```python
from build123d import *

# Parameters (mm, degrees)
RESSALTO_EXTRUS_O1_DEPTH            = 3
ESCAREADO_PARA_SFHCS_M31_AT_2_COUNT = 2
ESCAREADO_PARA_SFHCS_M31_AT_2_PITCH = 117.96437389
ESCAREADO_PARA_SFHCS_M31_AT_3_COUNT = 2
ESCAREADO_PARA_SFHCS_M31_AT_3_PITCH = 80
ESCAREADO_PARA_SFHCS_M31_AT_4_COUNT = 2
ESCAREADO_PARA_SFHCS_M31_AT_4_PITCH = 156.207361139
FILETE1_R                           = 4


with BuildPart() as part:
    # Esboço1 → Ressalto-extrusão1 (new body)
    with BuildSketch(Plane(origin=(0, 0, 0), x_dir=(1, 0, 0), z_dir=(0, 1, 0))):
        with BuildLine():
            Line((-68.089865002, 52.533515816), (-60.990156529, 50.415201884))
            Line((-60.990156529, 50.415201884), (-51.474506905, 61.094962266))
            Line((-51.474506905, 61.094962266), (-51.366345618, 68.974622419))
            ThreePointArc((-51.366345618, 68.974622419), (0, 86), (51.366345618, 68.974622419))
            Line((51.366345618, 68.974622419), (51.474506905, 61.094962266))
            Line((51.474506905, 61.094962266), (60.990156529, 50.415201884))
            Line((60.990156529, 50.415201884), (68.089865002, 52.533515816))
            ThreePointArc((68.089865002, 52.533515816), (85.999638052, 0.24950947), (68.393545574, -52.137538529))
            Line((68.393545574, -52.137538529), (60.990156529, -51.512941417))
            Line((60.990156529, -51.512941417), (50.318654012, -60.477268457))
            Line((50.318654012, -60.477268457), (51.474506905, -68.893941235))
            ThreePointArc((51.474506905, -68.893941235), (44.026252256, -73.876174185), (36.1, -78.056325817))
            Line((36.1, -78.056325817), (-36.1, -78.056325817))
            ThreePointArc((-36.1, -78.056325817), (-44.026252256, -73.876174185), (-51.474506905, -68.893941235))
            Line((-51.474506905, -68.893941235), (-50.318654012, -60.477268457))
            Line((-50.318654012, -60.477268457), (-60.990156529, -51.512941417))
            Line((-60.990156529, -51.512941417), (-68.393545574, -52.137538529))
            ThreePointArc((-68.393545574, -52.137538529), (-85.999638052, 0.24950947), (-68.089865002, 52.533515816))
        make_face()
    extrude(amount=RESSALTO_EXTRUS_O1_DEPTH)

    # Esboço3 → Escareado para SFHCS M31 (revolve, cut)
    with BuildSketch(Plane(origin=(40, 3, 69.282032303), x_dir=(0, 0, 1), z_dir=(1, 0, 0))):
        Polygon((0, 0), (0, 3), (1.7, 3), (1.7, 1.66), (3.36, 0), align=None)
    escareado_para_sfhcs_m31 = revolve(axis=Axis((40, 9.35, 69.282032303), (0, -1, 0)), mode=Mode.SUBTRACT)

    # Escareado para SFHCS M31 at 2: Escareado para SFHCS M31 ×2
    with Locations(*[Vector(0.21643961393810332, 0, -0.9762960071199333) * (i * ESCAREADO_PARA_SFHCS_M31_AT_2_PITCH) for i in range(1, ESCAREADO_PARA_SFHCS_M31_AT_2_COUNT)]):
        add(escareado_para_sfhcs_m31, mode=Mode.SUBTRACT)

    # Escareado para SFHCS M31 at 3: Escareado para SFHCS M31 ×2
    with Locations(*[(-i * ESCAREADO_PARA_SFHCS_M31_AT_3_PITCH, 0, 0) for i in range(1, ESCAREADO_PARA_SFHCS_M31_AT_3_COUNT)]):
        add(escareado_para_sfhcs_m31, mode=Mode.SUBTRACT)

    # Escareado para SFHCS M31 at 4: Escareado para SFHCS M31 ×2
    with Locations(*[Vector(-0.6755902076156564, 0, -0.7372773368101276) * (i * ESCAREADO_PARA_SFHCS_M31_AT_4_PITCH) for i in range(1, ESCAREADO_PARA_SFHCS_M31_AT_4_COUNT)]):
        add(escareado_para_sfhcs_m31, mode=Mode.SUBTRACT)

    # Filete1
    filete1_edges = [part.edges().sort_by_distance(p)[0] for p in [
        (-68.089865002, 1.5, -52.533515816),
        (-60.990156529, 1.5, -50.415201884),
        (-51.474506905, 1.5, -61.094962266),
        (-51.366345618, 1.5, -68.974622419),
        (51.366345618, 1.5, -68.974622419),
        (51.474506905, 1.5, -61.094962266),
        (60.990156529, 1.5, -50.415201884),
        (68.089865002, 1.5, -52.533515816),
        (68.393545574, 1.5, 52.137538529),
        (60.990156529, 1.5, 51.512941417),
        (50.318654012, 1.5, 60.477268457),
        (51.474506905, 1.5, 68.893941235),
        (-51.474506905, 1.5, 68.893941235),
        (-50.318654012, 1.5, 60.477268457),
        (-60.990156529, 1.5, 51.512941417),
        (-68.393545574, 1.5, 52.137538529),
    ]]
    fillet(filete1_edges, radius=FILETE1_R)


solid = part.part
```
CAD build for the part. Positions are in the model's coordinates, mm. Round coordinates to 2 decimals unless told otherwise and drop trailing zeros. Loops run counter-clockwise (first coordinate to the right, second up) from the corner with the lowest first, then second, coordinate; pieces in that order, holes last. Notation, with made-up numbers: M -18,46 L 26,46 A30 ccw 26,80 Z; hole C -38,10 d1. An arc over 180 degrees is marked long. Use a Markdown table: item, result. Add a question column.
(1) Drill centre lines: line 1 (X direction, y = 1.1, z = 70.5); line 2 (X direction, y = 0.8, z = -60); line 3 (X direction, y = 2.5, z = 60). Where is each one in solid material? Low to high.
(2) Cut at C-C (z = -65). Give the cut face in (x, y), and give its area (3 significant figures).
(3) Cut at A-A (z = -17). Give the cut face in (x, y).
(4) Flat gauge pins, fed straight in: pin 1 (3 mm diameter, centred on x = 65.53, z = -45.89, fed in from +Y); pin 2 (1.5 mm diameter, centred on x = -51, y = 1, fed in from +Z); pin 3 (5.5 mm diameter, centred on x = -65.53, z = -45.89, fed in from +Y). Where does each tip first touch, or does it go through?
(5) Cut at B-B (y = 0.45). State how many separate pieces and enclosed holes the cut face has, and give its area (3 significant figures).
Geometry says:
| question | item | result |
|---|---|---|
| 1 | line 1 | x = -49.25 to -41.19, -38.81 to 38.81, 41.19 to 49.25 |
| 1 | line 2 | x = -52.45 to 52.45 |
| 1 | line 3 | x = -51.19 to 51.19 |
| 2 | outline | M -51.42,0 L 51.42,0 L 51.42,3 L -51.42,3 Z |
| 2 | area | 309 mm² |
| 3 | outline | M -84.3,0 L 84.3,0 L 84.3,3 L -84.3,3 Z |
| 4 | pin 1 | passes through |
| 4 | pin 2 | stops at z = 69.63 |
| 4 | pin 3 | stops at y = 2.39 |
| 5 | separate pieces | 1 |
| 5 | enclosed holes | 4 |
| 5 | area | 22,300 mm² |
